The model under review builds one solid part; all positions refer to its coordinate system, in mm. A direction names the side the tool comes from. Coordinates: 2 decimals unless noted, no trailing zeros. Write each loop counter-clockwise with the first axis right and the second up, starting at its lowest first coordinate (ties: lowest second). Pieces come first, ordered by that corner, then holes.
Autodesk Inventor part; units mm, degrees
ref_plane "YZ Plane" through (0, 0, 0) normal (1, 0, 0) x (0, 1, 0)
ref_plane "XZ Plane" through (0, 0, 0) normal (0, 1, 0) x (-1, 0, 0)
ref_plane "XY Plane" through (0, 0, 0) normal (0, 0, 1) x (1, 0, 0)
sketch "Sketch1" plane through (0, 0, 0) normal (0, 0, 1) x (1, 0, 0)
  circle A0 centre (0, 0) radius 90
  circle A1 centre (0, 0) radius 10
  dimension "d1" = 20
  dimension "d2" = 180
extrude "Extrusion1" add sketch "Sketch1" along normal blind 15
sketch "Sketch2" plane through (0, 0, 15) normal (0, 0, 1) x (1, 0, 0)
  circle A0 centre (0, 55) radius 25
  circle A1 centre (-47.6314, 27.5) radius 25
  circle A2 centre (-47.6314, -27.5) radius 25
  circle A3 centre (0, -55) radius 25
  circle A4 centre (47.6314, -27.5) radius 25
  circle A5 centre (47.6314, 27.5) radius 25
  circle A6 centre (0, 55) radius 15
  circle A7 centre (-47.6314, 27.5) radius 15
  circle A8 centre (-47.6314, -27.5) radius 15
  circle A9 centre (0, -55) radius 15
  circle A10 centre (47.6314, -27.5) radius 15
  circle A11 centre (47.6314, 27.5) radius 15
  point P0 (0, 0)
  point P1 (0, 0)
  point P2 (0, 0)
  point P3 (0, 0)
  point P4 (0, 0)
  point P5 (0, 0)
  dimension "d5" = 50
  dimension "d6" = 55
  dimension "d9" = 360
  dimension "d11" = 30
  dimension "d14" = 360
extrude "Extrusion2" cut sketch "Sketch2" against normal blind 15 contours A6 | A7 | A8 | A9 | A10 | A11
sketch "Sketch3" plane through (0, 0, 15) normal (0, 0, 1) x (1, 0, 0)
  circle A0 centre (0, 0) radius 90
  circle A1 centre (0, 0) radius 80
  dimension "d18" = 160
  dimension "d19" = 180
extrude "Extrusion3" add sketch "Sketch3" along normal blind 100
sketch "Sketch4" plane through (0, 0, 15) normal (0, 0, 1) x (1, 0, 0)
  circle A0 centre (0, -54.6919) radius 25
  circle A1 centre (47.3646, -27.3459) radius 25
  circle A2 centre (47.3646, 27.3459) radius 25
  circle A3 centre (0, 54.6919) radius 25
  circle A4 centre (-47.3646, 27.3459) radius 25
  circle A5 centre (-47.3646, -27.3459) radius 25
  circle A6 centre (0, 0) radius 17.5
  circle A7 centre (0, 0) radius 10
  dimension "d22" = 50
  dimension "d25" = 360
  dimension "d27" = 35
extrude "Extrusion4" add sketch "Sketch4" along normal blind 100 contours A6 | A7
sketch "Sketch5" plane through (0, 0, 115) normal (0, 0, 1) x (1, 0, 0)
  circle A0 centre (0, 0) radius 10
  dimension "d30" = 20
extrude "Extrusion5" cut sketch "Sketch5" against normal through all
sketch "Sketch8" plane through (0, 0, 115) normal (0, 0, 1) x (1, 0, 0)
  point P0 (0, 0)
  point P1 (0, 85)
  point P2 (0, -85)
  dimension "d37" = 85
  dimension "d38" = 85
hole "Hole1" at (0, 85, 115) at (0, -85, 115) direction (0, 0, -1) diameter 3.4587 depth 10.8 tip angle 118
equation "\"BendRadius\" = Thickness"
equation "\"BendReliefWidth\" = Thickness"
equation "\"BendReliefDepth\" = 0.5 * Thickness"
equation "\"CornerReliefSize\" = 4 * Thickness"
equation "\"MinimumRemnant\" = 2 * Thickness"
equation "\"TransitionRadius\" = BendRadius"
equation "\"JacobiRadiusSize\" = BendRadius"
equation "\"GapSize\" = Thickness"
properties part number "Electromagnet cover"
Item 1: Mouldability with a two-part tool opening along Y and no side actions: class faces 3 (the face through (61.488, 21.755, 7.605)), 4 (the face through (41.53, 79.845, 56.695)), 5 (the face through (8, -8, 115)) as pulls with the +Y half, pulls with the -Y half, needs draft (parallel to the pull), parting line crosses it, or undercut.
Solved:
face 3: undercut
face 4: parting line crosses it
face 5: needs draft
Item 2: Take a section at D-D, the plane x = -27. Write out the cut boundary in (y, z).
Solved:
outline: (-85.85, 0) - (85.85, 0) - (85.85, 115) - (75.31, 115) - (75.31, 15) - (-75.31, 15) - (-75.31, 115) - (-85.85, 115) - close
Item 3: Machinability: for faces 1 (the face through (-3.252, 40.357, 7.605)), 2 (the face through (-17.34, 78.1, 64.3)), which of the approach directions +Z, -Z, +X, -X, +Y, -Y give a long, thin tool a straight path to every point of the face, cutting with its end or side? Answer none if there is none.
Solved:
face 1: +Z, -Z
face 2: +Z
Item 4: To check wall thickness, follow line 1 along Y through (x, z) = (0, 90); line 2 along X through (y, z) = (-5, 31.5); line 3 along X through (y, z) = (27, 5). State the ranges of each line that lie inside material, in increasing order.
Solved:
line 1: y = -90 to -80, -17.5 to -10, 10 to 17.5, 80 to 90
line 2: x = -89.86 to -79.84, -16.77 to -8.66, 8.66 to 16.77, 79.84 to 89.86
line 3: x = -85.85 to -62.62, -32.64 to 32.64, 62.62 to 85.85
Item 5: For pin 1 (4 mm diameter, centred on y = -55.5, z = 75.5, fed in from -X); pin 2 (3 mm diameter, centred on x = 0, y = 85, fed in from +Z); pin 3 (24 mm diameter, centred on x = 47.63, y = 27.5, fed in from +Z); pin 4 (2 mm diameter, centred on x = 21.5, z = 79, fed in from -Y), all flat-tipped, find the tip position at first contact; note any pin that passes through.
Solved:
pin 1: stops at x = -72.37
pin 2: stops at z = 104.06
pin 3: passes through
pin 4: stops at y = -87.63
Item 6: Take a section at A-A, the plane y = 0. Write out the cut boundary in (x, z), plus the area to 3 significant figures.
Solved:
outline: (-90, 0) - (-10, 0) - (-10, 115) - (-17.5, 115) - (-17.5, 15) - (-80, 15) - (-80, 115) - (-90, 115) - close; (10, 0) - (90, 0) - (90, 115) - (80, 115) - (80, 15) - (17.5, 15) - (17.5, 115) - (10, 115) - close
area: 5,900 mm2
Item 7: Take a section at C-C, the plane x = 47. Write out the cut boundary in (y, z).
Solved:
outline: (-76.75, 0) - (-42.49, 0) - (-42.49, 15) - (-64.74, 15) - (-64.74, 115) - (-76.75, 115) - close; (-12.51, 0) - (12.51, 0) - (12.51, 15) - (-12.51, 15) - close; (42.49, 0) - (76.75, 0) - (76.75, 115) - (64.74, 115) - (64.74, 15) - (42.49, 15) - close
Item 8: Take a section at B-B, the plane z = 100.5. Write out the cut boundary in (x, y), plus the area to 3 significant figures.
Solved:
outline: circle Ø180 at (0, 0); circle Ø35 at (0, 0); hole circle Ø160 at (0, 0); hole circle Ø20 at (0, 0)
area: 5,990 mm2
